Check sheet for the modelled part. Datum: model origin and axes. Units: mm. Round coordinates to 2 decimals unless told otherwise and drop trailing zeros. Write each loop counter-clockwise with the first axis right and the second up, starting at its lowest first coordinate (ties: lowest second). Pieces come first, ordered by that corner, then holes. Notation, with made-up numbers: (58, 54.5) - (62, 54.5) arc R24 ccw to (62, 87.5) - close; hole circle Ø5 at (50.5, 70). An arc over 180 degrees is marked (long way). Use one line per item in the form item = value. Start each with the question number.
1) Scan lines: probe 1 along Z at (x, y) = (-42, 0.3); probe 2 along Z at (x, y) = (8.5, 2); probe 3 along X at (y, z) = (0.7, -63.5). Record each from-to range of solid material in increasing order.
2) Section check A-A (z = 11.5). Record the boundary of the cut face in (x, y), then the cut area to 3 significant figures.
3) Section check B-B (y = 0.8). Count the separate pieces of the cut face and the enclosed holes in it, then the cut area to 3 significant figures.
4) Gauge pin test, flat ends, axial feed: P1, Ø1.9, axis at x = 8.23, z = -54.45, coming from the -Y side; P2, Ø4, axis at x = -60.27, z = 20.21, coming from the -Y side; P3, Ø1, axis at y = 0.5, z = -72.5, coming from the -X side. Record the tip position at first contact, or that the pin passes through.
5) Section check C-C (x = 2). Record the boundary of the cut face in (y, z), then the cut area to 3 significant figures.
from build123d import *

# Parameters (mm, degrees)
SKETCH1_R           = 1.6
BOSS_EXTRUDE1_DEPTH = 2.3
FILLET1_R           = 3
SKETCH3_R           = 4
CUT_EXTRUDE1_DEPTH  = 44.3
FILLET2_R           = 3


with BuildPart() as part:
    # Sketch1 → Boss-Extrude1 (new body)
    with BuildSketch(Plane(origin=(0, 0, 0), x_dir=(1, 0, 0), z_dir=(0, 1, 0))):
        with BuildLine():
            Line((18.815976516, 65.132242613), (2.251488694, 74.439107992))
            Line((2.251488694, 74.439107992), (8.509906392, 85.577926437))
            ThreePointArc((8.509906392, 85.577926437), (-43.86830382, 73.970074489), (-79.174773721, 33.576110647))
            Line((-79.174773721, 33.576110647), (-66.399065131, 33.725571155))
            Line((-66.399065131, 33.725571155), (-65.732278943, -23.270528678))
            Line((-65.732278943, -23.270528678), (-17.85230327, -22.710390238))
            Line((-17.85230327, -22.710390238), (-18.111073304, -0.591031778))
            Line((-18.111073304, -0.591031778), (18.815976516, 65.132242613))
        make_face()
        with Locations(Location((12.634623312, 62.296599376, 0), (0, 0, 270))):
            Circle(SKETCH1_R, mode=Mode.SUBTRACT)
        with Locations(Location((8.226108132, 54.450263039, 0), (0, 0, 270))):
            Circle(SKETCH1_R, mode=Mode.SUBTRACT)
        with Locations(Location((-42.268980916, -19.995830873, 0), (0, 0, 270))):
            Circle(SKETCH1_R, mode=Mode.SUBTRACT)
        with Locations(Location((-60.267749285, -20.206394932, 0), (0, 0, 270))):
            Circle(SKETCH1_R, mode=Mode.SUBTRACT)
        with Locations(Location((-55.633474662, 61.59477654, 0), (0, 0, 270))):
            Circle(SKETCH1_R, mode=Mode.SUBTRACT)
    extrude(amount=BOSS_EXTRUDE1_DEPTH)

    # Fillet1
    fillet1_edges = [part.edges().sort_by_distance(p)[0] for p in [
        (8.509906392, 1.15, -85.577926437),
        (2.251488694, 1.15, -74.439107992),
        (18.815976516, 1.15, -65.132242613),
        (-18.111073304, 1.15, 0.591031778),
        (-17.85230327, 1.15, 22.710390238),
        (-65.732278943, 1.15, 23.270528678),
        (-66.399065131, 1.15, -33.725571155),
        (-79.174773721, 1.15, -33.576110647),
    ]]
    fillet(fillet1_edges, radius=FILLET1_R)

    # Sketch3 → Cut-Extrude1 (cut)
    with BuildSketch(Plane(origin=(0, 2.3, 0), x_dir=(1, 0, 0), z_dir=(0, 1, 0))):
        with Locations((-30.257228913, 77.288421504)):
            Circle(SKETCH3_R)
        with Locations((-15.872582201, 81.468160248)):
            Circle(SKETCH3_R)
    extrude(amount=-CUT_EXTRUDE1_DEPTH, mode=Mode.SUBTRACT)

    # Fillet2
    fillet2_edges = [part.edges().sort_by_distance(p)[0] for p in [
        (-28.827983469, 1.15, -81.024362812),
        (-33.842999164, 1.15, -79.06106126),
        (-13.795112573, 1.15, -84.886364447),
        (-19.081339078, 1.15, -83.856439818),
    ]]
    fillet(fillet2_edges, radius=FILLET2_R)


solid = part.part
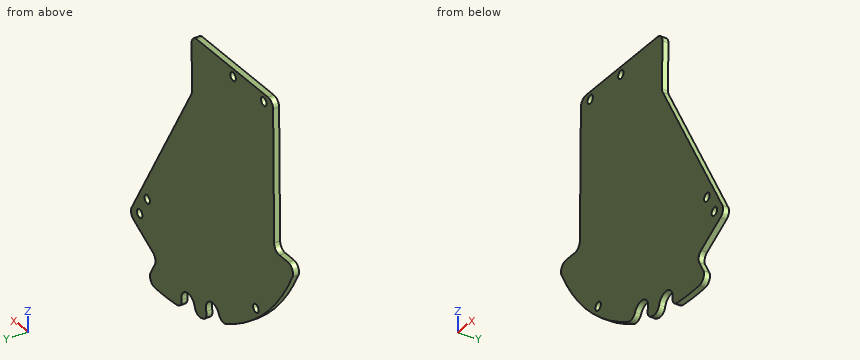
Results are:
q1.probe_1 = -75.05 to 18.42, 21.57 to 22.99
q1.probe_2 = -70.93 to -56.03, -52.87 to -46.77
q1.probe_3 = -58 to 11.58, 13.69 to 17.69
q2.outline = (-65.87, 0) - (-17.98, 0) - (-17.98, 2.3) - (-65.87, 2.3) - close
q2.area = 110 mm²
q3.separate_pieces = 1
q3.enclosed_holes = 5
q3.area = 6,350 mm²
q4.P1 = through
q4.P2 = 0
q4.P3 = -47.03
q5.outline = (0, -85.98) - (2.3, -85.98) - (2.3, -35.2) - (0, -35.2) - close
q5.area = 117 mm²
